Here's how the part is built. I have some questions about the finished solid (model axes, mm). Give positions to 0.01 mm unless a question says otherwise; leave off trailing zeros. Write each loop counter-clockwise with the first axis right and the second up, starting at its lowest first coordinate (ties: lowest second). Pieces come first, ordered by that corner, then holes. Notation, with made-up numbers: (-12.75, 22.25) - (24.25, 22.25) arc R25 cw to (24.25, 57.25) - close; hole circle Ø11 at (45.25, 11.5). An arc over 180 degrees is marked (long way). Use a Markdown table: item, result.
```python
from build123d import *

# Parameters (mm, degrees)
EXTRUDE3_DEPTH = 6.5
FILLET3_R      = 0.5
SKETCH2_R      = 4
EXTRUDE4_DEPTH = 6.5
FILLET5_R      = 0.5


with BuildPart() as part:
    # Sketch1 → Extrude3 (new body)
    with BuildSketch(Plane(origin=(0, 0, 0), x_dir=(1, 0, 0), z_dir=(0, 1, 0))):
        Polygon((7.5, 0), (3.75, 6.495190528), (-3.75, 6.495190528), (-7.5, 0), (-3.75, -6.495190528), (3.75, -6.495190528), align=None)
    extrude(amount=EXTRUDE3_DEPTH)

    # Fillet3
    fillet3_edges = [part.edges().sort_by_distance(p)[0] for p in [
        (0, 6.5, -6.495190528),
        (3.75, 3.25, 6.495190528),
        (-3.75, 3.25, 6.495190528),
        (-7.5, 3.25, 0),
        (-3.75, 3.25, -6.495190528),
        (3.75, 3.25, -6.495190528),
        (7.5, 3.25, 0),
        (-5.625, 6.5, -3.247595264),
        (-5.625, 6.5, 3.247595264),
        (0, 6.5, 6.495190528),
        (5.625, 6.5, 3.247595264),
        (0, 0, 6.495190528),
        (-5.625, 0, 3.247595264),
        (-5.625, 0, -3.247595264),
        (5.625, 6.5, -3.247595264),
        (0, 0, -6.495190528),
        (5.625, 0, -3.247595264),
        (5.625, 0, 3.247595264),
    ]]
    fillet(fillet3_edges, radius=FILLET3_R)

    # Sketch2 → Extrude4 (cut)
    with BuildSketch(Plane.XZ):
        Circle(SKETCH2_R)
    extrude(amount=-EXTRUDE4_DEPTH, mode=Mode.SUBTRACT)

    # Fillet5
    fillet5_edges = [part.edges().sort_by_distance(p)[0] for p in [
        (-4, 0, 0),
    ]]
    fillet(fillet5_edges, radius=FILLET5_R)


solid = part.part
```
Item 1: Thinking about a two-plate mould opening in X: for faces 1 (the cylindrical face through (-0.867, 3.458, -3.905)), 2 (the cylindrical face through (-5.477, 0.15, 3.218)), 3 (the flat face through (0, 3, -6.495)), 4 (the cylindrical face through (5.53, 0.15, 3.13)), which applies, +X half, -X half, draft (parallel to the pull), parting line (faces both ways), or undercut?
Values:
| item | result |
|---|---|
| face 1 | undercut |
| face 2 | -X half |
| face 3 | draft |
| face 4 | +X half |
Item 2: If we section it at B-B, the plane x = 0: Write out the boundary of the cut face in (y, z).
Values:
| item | result |
|---|---|
| outline | (0, -6) arc R0.5 ccw to (0.5, -6.5) - (6, -6.5) arc R0.5 ccw to (6.5, -6) - (6.5, -4) - (0.5, -4) arc R0.5 ccw to (0, -4.5) - close; (0, 4.5) arc R0.5 ccw to (0.5, 4) - (6.5, 4) - (6.5, 6) arc R0.5 ccw to (6, 6.5) - (0.5, 6.5) arc R0.5 ccw to (0, 6) - close |
Item 3: I need wall thicknesses on line 1 along Z through (x, y) = (0, 2.6); line 2 along Z through (x, y) = (1, 4.5); line 3 along X through (y, z) = (3.5, 1.25). Which ranges of each line are inside material? Lowest first, please. Write a range as [from, to].
Values:
| item | result |
|---|---|
| line 1 | z = [-6.5, -4], [4, 6.5] |
| line 2 | z = [-6.5, -3.87], [3.87, 6.5] |
| line 3 | x = [-6.78, -3.8], [3.8, 6.78] |
Item 4: Will these pins go through, and if not, where does the flat tip stop? pin 1 Ø3 at (y, z) = (4, 4.5) entering from +X; pin 2 Ø1.5 at (y, z) = (1, -1) entering from -X.
Values:
| item | result |
|---|---|
| pin 1 | stops at x = 5.77 |
| pin 2 | stops at x = -7.36 |
Item 5: If we section it at A-A, the plane y = 5: Write out the boundary of the cut face in (x, z).
Values:
| item | result |
|---|---|
| outline | (-7.36, -0.25) - (-3.89, -6.25) arc R0.5 ccw to (-3.46, -6.5) - (3.46, -6.5) arc R0.5 ccw to (3.89, -6.25) - (7.36, -0.25) arc R0.5 ccw to (7.36, 0.25) - (3.89, 6.25) arc R0.5 ccw to (3.46, 6.5) - (-3.46, 6.5) arc R0.5 ccw to (-3.89, 6.25) - (-7.36, 0.25) arc R0.5 ccw to start; hole circle Ø8 at (0, 0) |
